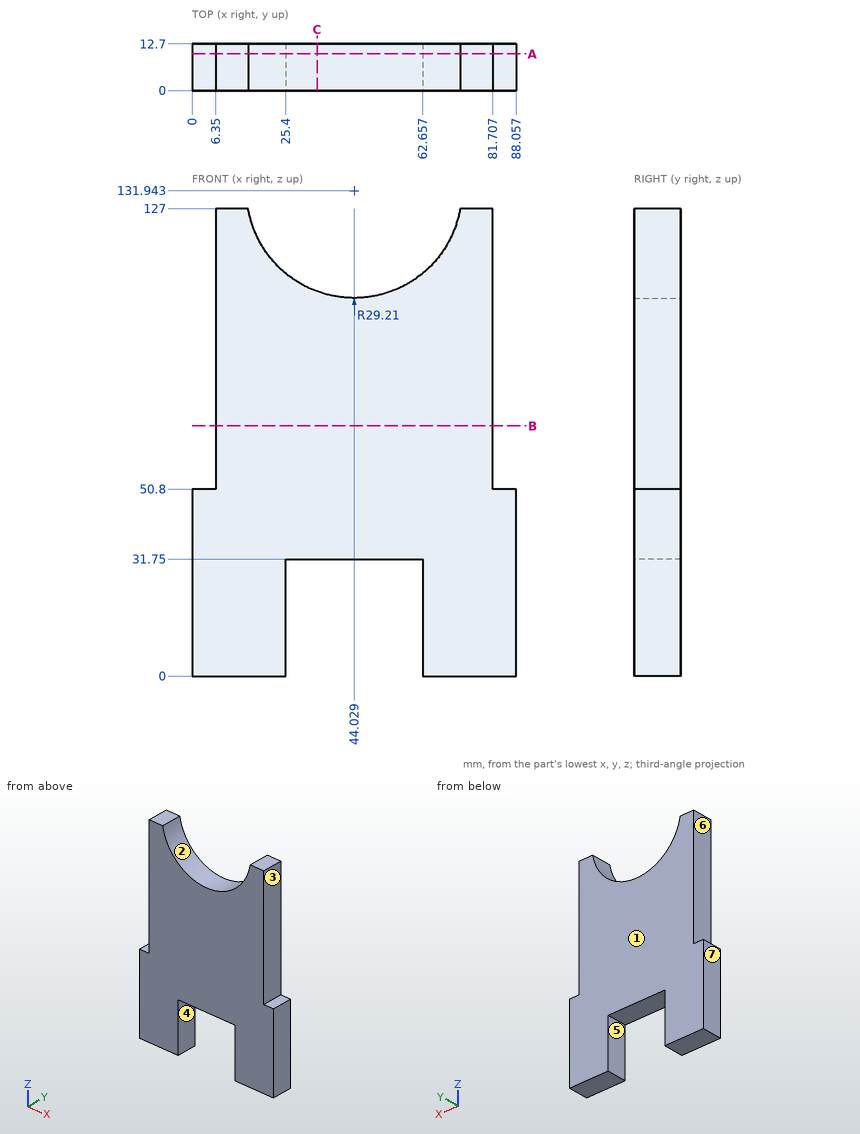
The figure shows three views and two pictorial views of one solid part (mm, origin at its lowest corner). Answer the questions. A direction names the side the tool comes from. Give positions to 0.01 mm unless a question says otherwise; leave off trailing zeros. Order: outer loops, then holes, each group sorted by start corner. A loop starts at its lowest first (then second) coordinate and runs counter-clockwise, first axis right, second up. Notation, with made-up numbers: (-32.75, 36.25) -> (8.25, 36.25) arc R25 ccw to (8.25, 50.25) -> close; hole circle Ø3 at (-6.75, 81.25). An arc over 180 degrees is marked (long way). Answer as CSV lines item,"result". Start each with the question number.
(1) Each of these flat-tipped pins is pushed along its axis until it touches: pin 1 Ø3 at (x, y) = (83.5, 9) entering from +Z; pin 2 Ø6.5 at (y, z) = (8, 100.5) entering from -X; pin 3 Ø6 at (x, y) = (61, 7) entering from +Z. Where does it stop, or does it pass through?
(2) For a pull along X with two mould halves and no side action, classify the marked faces 1, 2, 3 and 4 as released by +X, released by -X, zero draft, split by the parting line, or undercut.
(3) Consider line 1 along Z through (x, y) = (43.5, 11.75); line 2 along X through (y, z) = (10.25, 65); line 3 along Z through (x, y) = (4, 5.5). Determine where each line is inside the solid, lowest interval first.
(4) Section A-A, the plane y = 10 is taken. Write down the section's boundary in (x, z), plus the area to 3 significant figures.
(5) Which of the six approach directions +Z, -Z, +X, -X, +Y, -Y give full straight-line access (tool end or side, diameter ignored) to the marked faces 5, 6 and 7?
(6) Section C-C, the plane x = 34 is taken. Write down the section's boundary in (y, z).
(7) Section B-B, the plane z = 68 is taken. Write down the section's boundary in (x, y), plus the area to 3 significant figures.
Entries:
1,pin 1,"z = 50.8"
1,pin 2,"x = 6.35"
1,pin 3,"z = 110.63"
2,face 1,"zero draft"
2,face 2,"undercut"
2,face 3,"released by +X"
2,face 4,"undercut"
3,line 1,"31.75 to 102.74"
3,line 2,"6.35 to 81.71"
3,line 3,"0 to 50.8"
4,outline,"(0, 0) -> (25.4, 0) -> (25.4, 31.75) -> (62.66, 31.75) -> (62.66, 0) -> (88.06, 0) -> (88.06, 50.8) -> (81.71, 50.8) -> (81.71, 127) -> (72.82, 127) arc R29.21 cw to (15.24, 127) -> (6.35, 127) -> (6.35, 50.8) -> (0, 50.8) -> close"
4,area,"7,980 mm²"
5,face 5,"-Z, +Y, -Y"
5,face 6,"+Z, -X, +Y, -Y"
5,face 7,"+Z, -Z, -X, +Y, -Y"
6,outline,"(0, 31.75) -> (12.7, 31.75) -> (12.7, 104.51) -> (0, 104.51) -> close"
7,outline,"(6.35, 0) -> (81.71, 0) -> (81.71, 12.7) -> (6.35, 12.7) -> close"
7,area,"957 mm²"
